```python
from build123d import *

# Parameters (mm, degrees)
CUT_EXTRUDE1_DEPTH      = 1
CUT_EXTRUDE1_DEPTH_BACK = 16.875


with BuildPart() as part:
    # Sketch2 → Revolve1 (revolve)
    with BuildSketch(Plane(origin=(0, 0, 0), x_dir=(0, 0, -1), z_dir=(1, 0, 0))):
        Polygon((2.54, -3.2131), (8.89, -3.2131), (8.89, -3.4671), (25.5016, -3.4671), (25.5016, -5.8166), (22.9235, -5.8166), (22.9235, -16.4846), (25.5016, -16.4846), (25.5016, -18.8341), (8.89, -18.8341), (8.89, -19.0881), (2.54, -19.0881), align=None)
    revolve(axis=Axis((0, 55, 0), (0, -1, 0)))

    # Sketch3 → Cut-Extrude1 (cut, two sides)
    with BuildSketch(Plane(origin=(0, -3.2131, 0), x_dir=(1, 0, 0), z_dir=(0, 1, 0))) as cut_extrude1_sk:
        Polygon((3.695503603, 6.4008), (-3.695503603, 6.4008), (-7.391007206, 0), (-3.695503603, -6.4008), (3.695503603, -6.4008), (7.391007206, 0), align=None)
    extrude(amount=CUT_EXTRUDE1_DEPTH, mode=Mode.SUBTRACT)
    extrude(cut_extrude1_sk.sketch, amount=-CUT_EXTRUDE1_DEPTH_BACK, mode=Mode.SUBTRACT)


solid = part.part
```
Geometry: final body of the model. Coordinates: model frame, mm. A direction names the side the tool comes from. Coordinates: 2 decimals unless noted, no trailing zeros. Order: outer loops, then holes, each group sorted by start corner. A loop starts at its lowest first (then second) coordinate and runs counter-clockwise, first axis right, second up. Notation, with made-up numbers: (41, -38.5) -> (63, -38.5) arc R4 ccw to (63, -34.5) -> close; hole circle Ø3 at (-6, 8). An arc over 180 degrees is marked (long way). Use CSV: the item, a comma, the result in double quotes.
1) Section A-A on x = 0. Output: boundary loops of the cut face in (y, z).
Findings:
outline,"(-19.09, -8.89) -> (-18.83, -8.89) -> (-18.83, -25.5) -> (-16.48, -25.5) -> (-16.48, -22.92) -> (-5.82, -22.92) -> (-5.82, -25.5) -> (-3.47, -25.5) -> (-3.47, -8.89) -> (-3.21, -8.89) -> (-3.21, -6.4) -> (-19.09, -6.4) -> close; (-19.09, 6.4) -> (-3.21, 6.4) -> (-3.21, 8.89) -> (-3.47, 8.89) -> (-3.47, 25.5) -> (-5.82, 25.5) -> (-5.82, 22.92) -> (-16.48, 22.92) -> (-16.48, 25.5) -> (-18.83, 25.5) -> (-18.83, 8.89) -> (-19.09, 8.89) -> close"
2) Section C-C on z = 17. Output: boundary loops of the cut face in (x, y).
Findings:
outline,"(-19.01, -18.83) -> (19.01, -18.83) -> (19.01, -16.48) -> (15.38, -16.48) -> (15.38, -5.82) -> (19.01, -5.82) -> (19.01, -3.47) -> (-19.01, -3.47) -> (-19.01, -5.82) -> (-15.38, -5.82) -> (-15.38, -16.48) -> (-19.01, -16.48) -> close"
3) Mould query, pull axis Y, two halves, no side actions, for faces 1 (the cylindrical face through (-22.624, -4.658, -11.767)), 2 (the flat face through (10, -16.485, -21)), 3 (the flat face through (0, -18.834, -11)), 4 (the flat face through (10, -5.817, 21)). Classes: +Y half, -Y half, draft (parallel to the pull), parting line (faces both ways), or undercut.
Findings:
face 1,"draft"
face 2,"undercut"
face 3,"-Y half"
face 4,"undercut"
4) Line query: line 1 (Y direction, x = -16, z = 19.5); line 2 (Y direction, x = 11, z = -15.5); line 3 (X direction, y = -3.75, z = 6). Output: solid intervals per line, ascending.
Findings:
line 1,"y = -18.83 to -16.48, -5.82 to -3.47"
line 2,"y = -18.83 to -3.47"
line 3,"x = -24.79 to -3.93, 3.93 to 24.79"
5) Section B-B on y = -6.5. Output: boundary loops of the cut face in (x, z).
Findings:
outline,"circle Ø45.85 at (0, 0); hole (-7.39, 0) -> (-3.7, -6.4) -> (3.7, -6.4) -> (7.39, 0) -> (3.7, 6.4) -> (-3.7, 6.4) -> close"
6) Pin query (flat end, axial travel): pin 1 Ø3.5 at (x, y) = (1, -13) entering from -Z; pin 2 Ø5 at (x, y) = (8.5, -8.5) entering from +Z; pin 3 Ø5 at (x, y) = (19.5, -11.5) entering from +Z. Return the tip coordinate at first contact, or that it passes through.
Findings:
pin 1,"stops at z = -22.92"
pin 2,"stops at z = 22.12"
pin 3,"stops at z = 15.38"
7) Access query for faces 5 (the flat face through (5.569, -11.039, -3.156)), 6 (the cylindrical face through (22.73, -11.23, 2.98)), 7 (the flat face through (0, -3.467, 11)). Directions: +Z, -Z, +X, -X, +Y, -Y. A direction counts if a zero-diameter tool reaches every point of the face in a straight line with its end or side. Return the directions, or none.
Findings:
face 5,"+Y, -Y"
face 6,"none"
face 7,"+Y"
8) Section D-D on x = -11.5. Output: boundary loops of the cut face in (y, z), then the cut area to 3 significant figures.
Findings:
outline,"(-18.83, -22.76) -> (-16.48, -22.76) -> (-16.48, -19.83) -> (-5.82, -19.83) -> (-5.82, -22.76) -> (-3.47, -22.76) -> (-3.47, 22.76) -> (-5.82, 22.76) -> (-5.82, 19.83) -> (-16.48, 19.83) -> (-16.48, 22.76) -> (-18.83, 22.76) -> close"
area,"637 mm^2"
